CAD build for the part. Positions are in the model's coordinates, mm. Face numbers are marked on the shaded views. Round coordinates to 2 decimals unless told otherwise and drop trailing zeros. Loops run counter-clockwise (first coordinate to the right, second up) from the corner with the lowest first, then second, coordinate; pieces in that order, holes last. Notation, with made-up numbers: M 29.25,-12 L 64.25,-12 A12 ccw 64.25,-2 Z; hole C -4.75,63 d2. An arc over 180 degrees is marked long. Use one line per item in the form item = value.
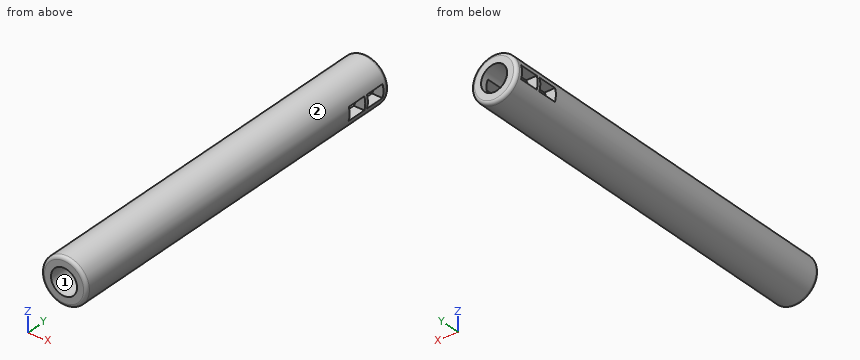
from build123d import *

# Parameters (mm, degrees)
F0_R     = 3.5
F0_R_2   = 2
F1_DEPTH = 58
F2_R     = 0.5
F3_W     = 3
F3_H     = 2
F4_DEPTH = 12.5


with BuildPart() as f1:
    # F0 (on Front) → F1 (new body)
    with BuildSketch(Plane.XZ):
        Circle(F0_R)
        Circle(F0_R_2, mode=Mode.SUBTRACT)
    extrude(amount=F1_DEPTH)

    # F2
    f2_edges = [f1.edges().sort_by_distance(p)[0] for p in [
        (-3.5, -58, 0),
        (-3.5, 0, 0),
    ]]
    fillet(f2_edges, radius=F2_R)

    # F3 (on Right) → F4 (cut, symmetric)
    with BuildSketch(Plane.YZ):
        with Locations((-6, 0)):
            Rectangle(F3_W, F3_H)
        with Locations((-2.5, 0)):
            Rectangle(F3_W, F3_H)
    extrude(amount=F4_DEPTH, both=True, mode=Mode.SUBTRACT)


solid = f1.part
1. Cut at A-A on x = 0. Write the cut outline in (y, z).
Completed:
outline = M -58,-3 A0.5 ccw -57.5,-3.5 L -0.5,-3.5 A0.5 ccw 0,-3 L 0,-2 L -58,-2 Z; M -58,2 L 0,2 L 0,3 A0.5 ccw -0.5,3.5 L -57.5,3.5 A0.5 ccw -58,3 Z
2. Pull direction X, two halves, no side cores. Call the marked faces 1 and 2: +X half, -X half, draft (parallel to the pull), parting line (faces both ways), or undercut.
Completed:
face_1 = undercut
face_2 = parting line
3. Drop flat-ended pins along their axis: P1, Ø1.5, axis at y = -25, z = -2.5, coming from the -X side; P2, Ø1.8, axis at x = 2.5, y = -6, coming from the -Z side; P3, Ø0.5, axis at x = 2.5, y = -5.5, coming from the +Z side. Give the stop position or say it passes through.
Completed:
P1 = -3.03
P2 = -3.11
P3 = 2.68
4. Cut at C-C on y = -41.5. Write the cut outline in (x, z), and give its area (3 significant figures).
Completed:
outline = C 0,0 d7; hole C 0,0 d4
area = 25.9 mm2
5. Probe line 1 along Z through (x, y) = (0, -32); line 2 along Y through (x, z) = (-0.5, -3). List the from-to ranges inside material, lowest first. Write a range as from..to.
Completed:
line_1 = -3.5..-2, 2..3.5
line_2 = -58..0
6. Cut at B-B on z = 0. Write the cut outline in (x, y).
Completed:
outline = M -3.5,-57.5 A0.5 ccw -3,-58 L -2,-58 L -2,-7.5 L -3.5,-7.5 Z; M -3.5,-4.5 L -2,-4.5 L -2,-4 L -3.5,-4 Z; M -3.5,-1 L -2,-1 L -2,0 L -3,0 A0.5 ccw -3.5,-0.5 Z; M 2,-58 L 3,-58 A0.5 ccw 3.5,-57.5 L 3.5,-7.5 L 2,-7.5 Z; M 2,-4.5 L 3.5,-4.5 L 3.5,-4 L 2,-4 Z; M 2,-1 L 3.5,-1 L 3.5,-0.5 A0.5 ccw 3,0 L 2,0 Z
7. Cut at D-D on x = 2.5. State how many separate pieces and enclosed holes the cut face has, and give its area (3 significant figures).
Completed:
separate_pieces = 1
enclosed_holes = 2
area = 272 mm2
